The listing builds one solid part. Answer for the finished solid, in the listing's coordinates (mm). A direction names the side the tool comes from. Coordinates: 2 decimals unless noted, no trailing zeros. Loops run counter-clockwise (first coordinate to the right, second up) from the corner with the lowest first, then second, coordinate; pieces in that order, holes last. Notation, with made-up numbers: (24.5, -39.75) -> (57.5, -39.75) arc R12 ccw to (57.5, -19.75) -> close; hole circle Ø6 at (-14.5, 57). An arc over 180 degrees is marked (long way). Answer in a Markdown table with one row per item.
```python
from build123d import *

# Parameters (mm, degrees)
SKETCH1_W           = 400
SKETCH1_H           = 500
BOSS_EXTRUDE1_DEPTH = 20
CUT_EXTRUDE2_DEPTH  = 473.122865365


with BuildPart() as part:
    # Sketch1 → Boss-Extrude1 (new body)
    with BuildSketch(Plane.XY):
        Rectangle(SKETCH1_W, SKETCH1_H)
    extrude(amount=BOSS_EXTRUDE1_DEPTH)

    # Sketch2 → Cut-Extrude2 (cut, through all)
    with BuildSketch(Plane(origin=(200, 0, 0), x_dir=(0, 0, -1), z_dir=(1, 0, 0))):
        Polygon((-1, 0), (-20.657237149, 19.657237149), (-20.657237149, -19.657237149), align=None)
    extrude(amount=-CUT_EXTRUDE2_DEPTH, mode=Mode.SUBTRACT)


solid = part.part
```
Item 1: A tool of negligible diameter and unlimited length cuts with its end or side. For faces 1 (the face through (3, 9, 10)), 2 (the face through (-3, 4, 0)), from which of +Z, -Z, +X, -X, +Y, -Y can it reach the whole face along a straight path? Write none if from no direction.
Findings below:
| item | result |
|---|---|
| face 1 | +Z, +X, -X |
| face 2 | -Z, +X, -X, +Y, -Y |
Item 2: A cutting plane is placed at A-A, the plane z = 9.25. Determine the outline of the cut face in (x, y), plus the area to 3 significant figures.
Findings below:
| item | result |
|---|---|
| outline | (-200, -250) -> (200, -250) -> (200, -8.25) -> (-200, -8.25) -> close; (-200, 8.25) -> (200, 8.25) -> (200, 250) -> (-200, 250) -> close |
| area | 193,000 mm2 |
Item 3: Find the intervals of material crossed by probe 1 along Y at (x, z) = (-27, 14.25); probe 2 along Y at (x, z) = (104, 5.5); probe 3 along Z at (x, y) = (-124, 18.5), in increasing order.
Findings below:
| item | result |
|---|---|
| probe 1 | y = -250 to -13.25, 13.25 to 250 |
| probe 2 | y = -250 to -4.5, 4.5 to 250 |
| probe 3 | z = 0 to 19.5 |
Item 4: A cutting plane is placed at C-C, the plane y = -8. Determine the outline of the cut face in (x, z), plus the area to 3 significant figures.
Findings below:
| item | result |
|---|---|
| outline | (-200, 0) -> (200, 0) -> (200, 9) -> (-200, 9) -> close |
| area | 3,600 mm2 |
Item 5: A cutting plane is placed at B-B, the plane x = -110. Determine the outline of the cut face in (y, z).
Findings below:
| item | result |
|---|---|
| outline | (-250, 0) -> (250, 0) -> (250, 20) -> (19, 20) -> (0, 1) -> (-19, 20) -> (-250, 20) -> close |
